Source: CAD feature listing. Evaluate the final solid. Frame: model axes, mm. Face numbers are marked on the shaded views. Coordinates: 2 decimals unless noted, no trailing zeros. Loops run counter-clockwise (first coordinate to the right, second up) from the corner with the lowest first, then second, coordinate; pieces in that order, holes last. Notation, with made-up numbers: M 33.25,56 L 42.25,56 A25 ccw 42.25,87 Z; hole C -6.75,76.5 d2. An arc over 180 degrees is marked long. One line per question, with ' | ' between items. Start each with the question number.
1. Section query B-B, the plane z = 16.5. Output: boundary loops of the cut face in (x, y), and give its area (3 significant figures).
2. Pin query (flat end, axial travel): P1, Ø4, axis at x = -10.5, z = 13.5, coming from the +Y side; P2, Ø4, axis at x = -7.5, z = 28, coming from the +Y side; P3, Ø8, axis at x = -7.5, z = 30, coming from the +Y side. Return the tip coordinate at first contact, or that it passes through.
3. Ray query, probe 1 along Z at (x, y) = (-12.7, 0.4) (1 decimal); probe 2 along Z at (x, y) = (3, 8.5) (3 decimals); probe 3 along X at (y, z) = (3, 19.5). Return the intervals inside material, ascending.
4. Section query D-D, the plane z = 31.5. Output: boundary loops of the cut face in (x, y), and give its area (3 significant figures).
5. Mould query, pull axis X, two halves, no side actions, for the marked faces 1 and 2. Classes: pulls with the +X half, pulls with the -X half, needs draft (parallel to the pull), parting line crosses it, or undercut.
6. Section query C-C, the plane y = 1.5. Output: boundary loops of the cut face in (x, z) (3 decimals), and give its area (3 significant figures).
7. Section query A-A, the plane x = 12.7. Output: boundary loops of the cut face in (y, z) (1 decimal).
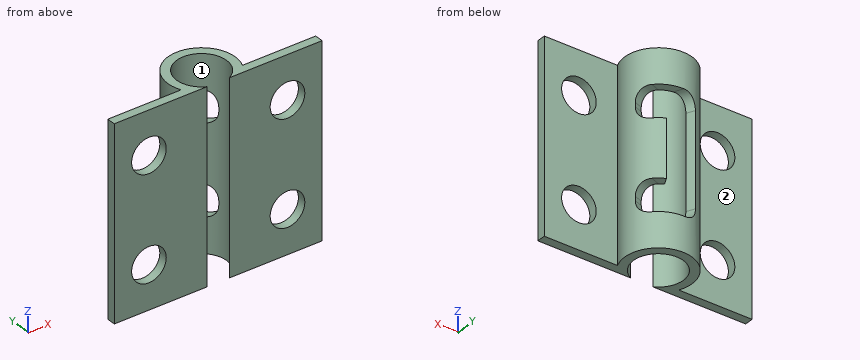
```python
from build123d import *

# Parameters (mm, degrees)
F1_DEPTH  = 34.925
F3_D      = 6.35
F6_DEPTH  = 22.225
F8_DEPTH  = 5.842
F10_DEPTH = 5.842
F11_R     = 2.54


with BuildPart() as f1:
    # F0 (on Top) → F1 (new body)
    with BuildSketch(Plane.XY):
        with BuildLine():
            Line((-5.6265138051, 0.79375), (-19.05, 0.79375))
            Line((-19.05, 0.79375), (-19.05, -0.79375))
            Line((-19.05, -0.79375), (-2.035580681, -0.79375))
            ThreePointArc((-2.035580681, -0.79375), (0, 7.8720984695), (2.035580681, -0.79375))
            Line((2.035580681, -0.79375), (19.05, -0.79375))
            Line((19.05, -0.79375), (19.05, 0.79375))
            Line((19.05, 0.79375), (5.6265138051, 0.79375))
            ThreePointArc((5.6265138051, 0.79375), (0, 9.4595984695), (-5.6265138051, 0.79375))
        make_face()
    extrude(amount=F1_DEPTH)

    # F3 (through all)
    with Locations(Plane(origin=(0, 0.79375, 0), x_dir=(-1, 0, 0), z_dir=(0, 1, 0))):
        with Locations((12.7, 7.9375), (12.7, 26.9875), (-12.7, 26.9875), (-12.7, 7.9375)):
            Hole(F3_D / 2)

    # F5 (on offset) → F6 (cut)
    with BuildSketch(Plane.XY.offset(6.35)):
        Polygon((-4.318, 12.3874302953), (0, 3.3000984695), (4.318, 12.3874302953), align=None)
    extrude(amount=F6_DEPTH, mode=Mode.SUBTRACT)

    # F7 (on offset) → F8 (cut)
    with BuildSketch(Plane.XY.offset(6.35)):
        Polygon((0, 15.2833266184), (0, 3.3000984695), (13.4768653661, 8.1709222868), align=None)
    extrude(amount=F8_DEPTH, mode=Mode.SUBTRACT)

    # F9 (on face) → F10 (cut)
    with BuildSketch(Plane(origin=(0, 0, 28.575), x_dir=(1, 0, 0), z_dir=(0, 0, -1))):
        Polygon((8.5841133563, -6.4025783601), (0, -3.3000984695), (0, -13.6242890731), align=None)
    extrude(amount=F10_DEPTH, mode=Mode.SUBTRACT)

    # F11
    f11_edges = [f1.edges().sort_by_distance(p)[0] for p in [
        (-2.302872, 8.146546, 28.575),
        (-2.302872, 8.146546, 6.35),
        (5.046277, 5.12393, 6.35),
        (5.046277, 5.12393, 12.192),
        (5.046277, 5.12393, 22.733),
        (5.046277, 5.12393, 28.575),
    ]]
    fillet(f11_edges, radius=F11_R)


solid = f1.part
```
Taken from the geometry:
1) outline: M -19.05,-0.79 L -2.04,-0.79 A4.57 cw -1.96,7.43 L -2.64,8.86 A6.16 ccw -5.63,0.79 L -19.05,0.79 Z; M 1.96,7.43 A4.57 cw 2.04,-0.79 L 19.05,-0.79 L 19.05,0.79 L 5.63,0.79 A6.16 ccw 2.64,8.86 Z | area: 78.2 mm^2
2) P1: y = 0.79 | P2: y = 6.07 | P3: y = 8.37
3) probe 1: 0 to 4.8, 11.1 to 23.8, 30.2 to 34.9 | probe 2: 0 to 6.35, 12.192 to 22.733, 28.575 to 34.925 | probe 3: -6.15 to -4.56, 4.56 to 6.15
4) outline: M -19.05,-0.79 L -2.04,-0.79 A4.57 cw long 2.04,-0.79 L 19.05,-0.79 L 19.05,0.79 L 5.63,0.79 A6.16 ccw long -5.63,0.79 L -19.05,0.79 Z | area: 85.7 mm^2
5) face 1: undercut | face 2: needs draft
6) outline: M -5.891,0 L -4.203,0 L -4.203,34.925 L -5.891,34.925 Z; M 4.203,0 L 5.891,0 L 5.891,34.925 L 4.203,34.925 Z | area: 118 mm^2
7) outline: M -0.8,0 L 0.8,0 L 0.8,4.8 L -0.8,4.8 Z; M -0.8,11.1 L 0.8,11.1 L 0.8,23.8 L -0.8,23.8 Z; M -0.8,30.2 L 0.8,30.2 L 0.8,34.9 L -0.8,34.9 Z
